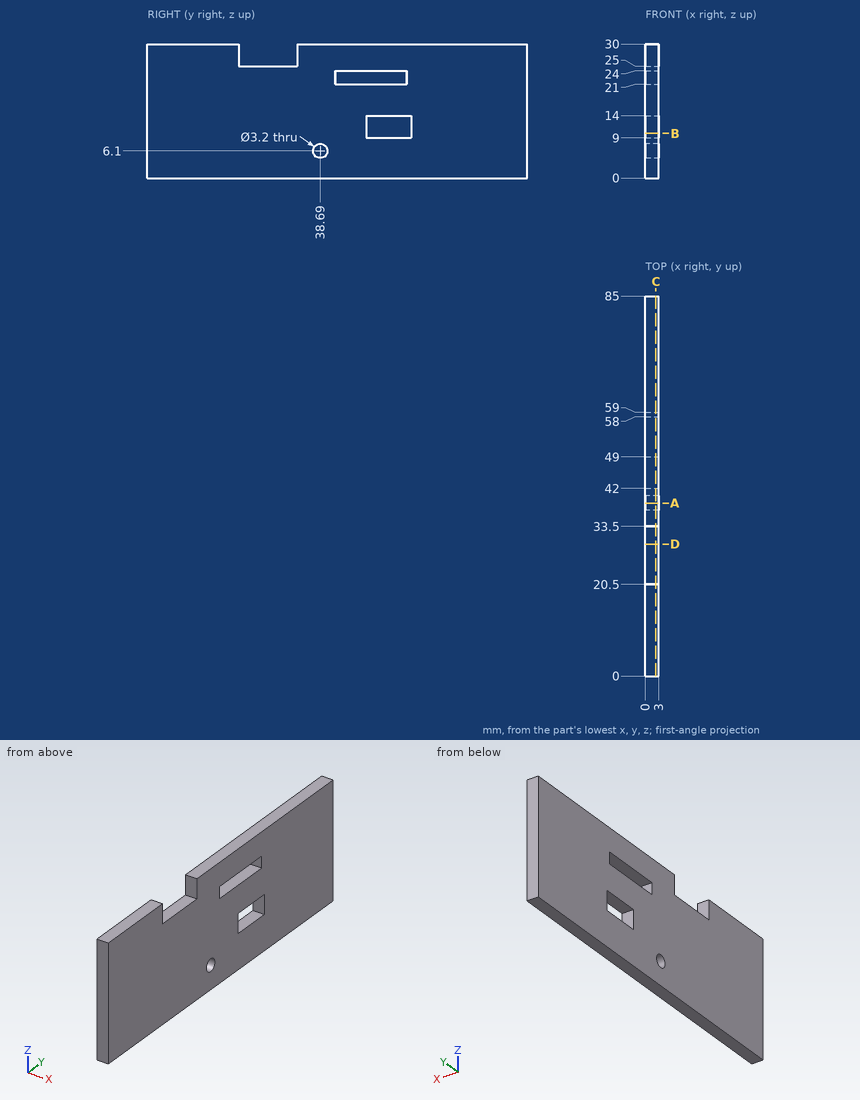
Geometry: see drawing. Coordinates: mm, zero at the bounding-box minimum. Coordinates: 2 decimals unless noted, no trailing zeros. Order: outer loops, then holes, each group sorted by start corner. A loop starts at its lowest first (then second) coordinate and runs counter-clockwise, first axis right, second up. Notation, with made-up numbers: M 81.5,62.5 L 121.5,62.5 A22 ccw 121.5,72.5 Z; hole C 46.25,-13.5 d5. An arc over 180 degrees is marked long. Write item = value, one per line. Start each with the question number.
(1) Section B-B on z = 10. Output: boundary loops of the cut face in (x, y), and give its area (3 significant figures).
(2) Line query: line 1 along Z through (x, y) = (1.65, 38.69); line 2 along Y through (x, z) = (0.7, 25.25); line 3 along Y through (x, z) = (0.9, 6.1). Output: solid intervals per line, ascending. Write a range as [from, to].
(3) Section D-D on y = 29.5. Output: boundary loops of the cut face in (x, z).
(4) Section C-C on x = 2.35. Output: boundary loops of the cut face in (y, z).
(5) Section A-A on y = 38.69. Output: boundary loops of the cut face in (x, z), and give its area (3 significant figures).
Result set:
q1.outline = M 0,0 L 3,0 L 3,49 L 0,49 Z; M 0,59 L 3,59 L 3,85 L 0,85 Z
q1.area = 225 mm²
q2.line_1 = [0, 4.5], [7.7, 30]
q2.line_2 = [0, 20.5], [33.5, 85]
q2.line_3 = [0, 37.09], [40.29, 85]
q3.outline = M 0,0 L 3,0 L 3,25 L 0,25 Z
q4.outline = M 0,0 L 85,0 L 85,30 L 33.5,30 L 33.5,25 L 20.5,25 L 20.5,30 L 0,30 Z; hole C 38.69,6.1 d3.2; hole M 42,21 L 58,21 L 58,24 L 42,24 Z; hole M 49,9 L 59,9 L 59,14 L 49,14 Z
q5.outline = M 0,0 L 3,0 L 3,4.5 L 0,4.5 Z; M 0,7.7 L 3,7.7 L 3,30 L 0,30 Z
q5.area = 80.4 mm²
